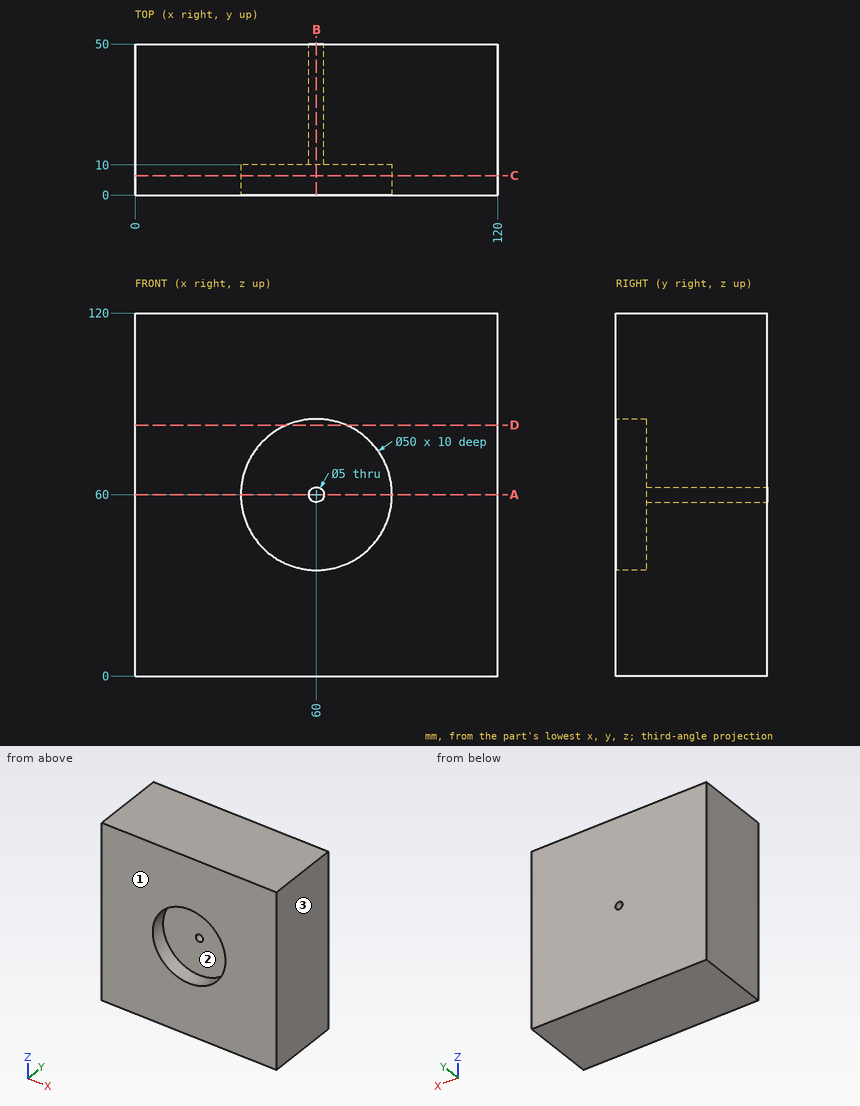
Source: three-view drawing plus pictorial views. Frame: mm from the lowest corner of the part. Coordinates: 2 decimals unless noted, no trailing zeros. Write each loop counter-clockwise with the first axis right and the second up, starting at its lowest first coordinate (ties: lowest second). Pieces come first, ordered by that corner, then holes. Notation, with made-up numbers: (66.5, -15) - (120.5, -15) arc R23 ccw to (120.5, 21) - close; hole circle Ø6 at (41.25, 1). An arc over 180 degrees is marked (long way). Return JSON: item names as keys, results as strings.
Item 1: Section query C-C (y = 6.5). Output: boundary loops of the cut face in (x, z).
Completed:
{"outline": "(0, 0) - (120, 0) - (120, 120) - (0, 120) - close; hole circle Ø50 at (60, 60)"}
Item 2: Section query B-B (x = 60). Output: boundary loops of the cut face in (y, z).
Completed:
{"outline": "(0, 0) - (50, 0) - (50, 57.5) - (10, 57.5) - (10, 35) - (0, 35) - close; (0, 85) - (10, 85) - (10, 62.5) - (50, 62.5) - (50, 120) - (0, 120) - close"}
Item 3: Pull-direction query (X, two-part tool) for the marked faces 1, 2 and 3; classes: +X half, -X half, draft (parallel to the pull), parting line (faces both ways), or undercut.
Completed:
{"face 1": "draft", "face 2": "undercut", "face 3": "+X half"}
Item 4: Section query A-A (z = 60). Output: boundary loops of the cut face in (x, y), and give its area (3 significant figures).
Completed:
{"outline": "(0, 0) - (35, 0) - (35, 10) - (57.5, 10) - (57.5, 50) - (0, 50) - close; (62.5, 10) - (85, 10) - (85, 0) - (120, 0) - (120, 50) - (62.5, 50) - close", "area": "5,300 mm2"}
Item 5: Section query D-D (z = 83). Output: boundary loops of the cut face in (x, y), and give its area (3 significant figures).
Completed:
{"outline": "(0, 0) - (50.2, 0) - (50.2, 10) - (69.8, 10) - (69.8, 0) - (120, 0) - (120, 50) - (0, 50) - close", "area": "5,800 mm2"}
Item 6: Line query: L1, parallel to Z at x = 60, y = 19; L2, parallel to Z at x = 60, y = 4.25; L3, parallel to X at y = 3, z = 40.5. Output: solid intervals per line, ascending.
Completed:
{"L1": "z = 0 to 57.5, 62.5 to 120", "L2": "z = 0 to 35, 85 to 120", "L3": "x = 0 to 44.36, 75.64 to 120"}
